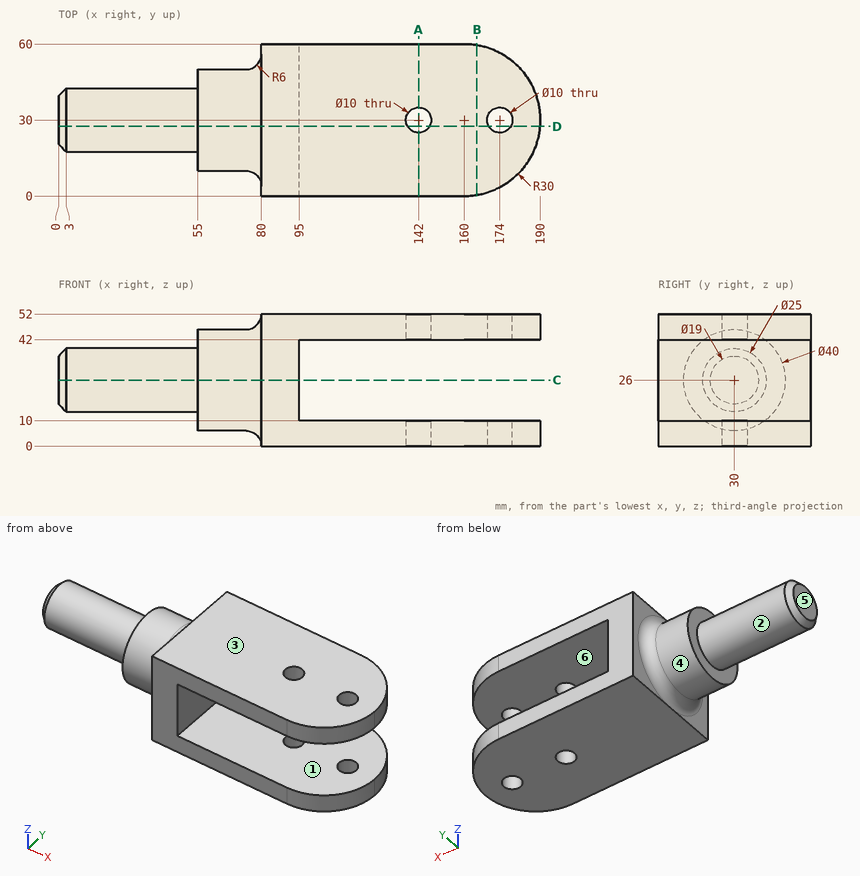
Design review of the part shown in the three views and the two pictorial views. Dimensions are in mm from the part's minimum x, y and z. A direction names the side the tool comes from. Round coordinates to 2 decimals unless told otherwise and drop trailing zeros. Write each loop counter-clockwise with the first axis right and the second up, starting at its lowest first coordinate (ties: lowest second). Pieces come first, ordered by that corner, then holes. Notation, with made-up numbers: (57, 47) - (110, 47) arc R25 cw to (110, 63) - close; hole circle Ø6 at (62.5, -23.75). An arc over 180 degrees is marked (long way). Write item = value, one per line. Start each with the question number.
1. Consider section D-D on y = 27.5. Give the number of separate pieces and of enclosed holes in the cut face, plus the area to 3 significant figures.
2. For the marked faces 1, 2 and 3, list the 3-axis set-ups (+Z, -Z, +X, -X, +Y, -Y) from which the entire face can be reached by the end or side of a thin tool; tool diameter is ignored.
3. Draft analysis for pull direction Z (two halves, no side actions). For the marked faces 4, 5 and 6, state which applies: released by +Z, released by -Z, zero draft, split by the parting line, or undercut.
4. Wall thickness on L1, parallel to X at y = 30, z = 45.75; L2, parallel to Z at x = 118, y = 19; L3, parallel to X at y = 30, z = 48: over which ranges is each line inside the solid? List them lowest first.
5. Consider section B-B on x = 165. State the section outline as (y, z) points, plus the area to 3 significant figures.
6. Consider section A-A on x = 142. State the section outline as (y, z) points.
7. For pin 1 Ø12 at (x, z) = (31, 16.5) entering from -Y; pin 2 Ø1.5 at (x, z) = (162, 5.5) entering from -Y; pin 3 Ø9.5 at (y, z) = (25.5, 30.5) entering from +X; pin 4 Ø10 at (x, z) = (125.5, 36.5) entering from +Y, all flat-tipped, find the tip position at first contact; note any pin that passes through.
8. Consider section C-C on z = 26. State the section outline as (x, y) points, plus the area to 3 significant figures.
Evaluation:
q1.separate_pieces = 5
q1.enclosed_holes = 0
q1.area = 4,680 mm2
q2.face_1 = +X, +Y, -Y
q2.face_2 = -X
q2.face_3 = +Z, +X, -X, +Y, -Y
q3.face_4 = split by the parting line
q3.face_5 = zero draft
q3.face_6 = undercut
q4.L1 = 55 to 137, 147 to 169, 179 to 190
q4.L2 = 0 to 10, 42 to 52
q4.L3 = 78.47 to 137, 147 to 169, 179 to 190
q5.outline = (0.42, 0) - (59.58, 0) - (59.58, 10) - (0.42, 10) - close; (0.42, 42) - (59.58, 42) - (59.58, 52) - (0.42, 52) - close
q5.area = 1,180 mm2
q6.outline = (0, 0) - (25, 0) - (25, 10) - (0, 10) - close; (0, 42) - (25, 42) - (25, 52) - (0, 52) - close; (35, 0) - (60, 0) - (60, 10) - (35, 10) - close; (35, 42) - (60, 42) - (60, 52) - (35, 52) - close
q7.pin_1 = 18
q7.pin_2 = 0.03
q7.pin_3 = 95
q7.pin_4 = through
q8.outline = (0, 20.5) - (3, 17.5) - (55, 17.5) - (55, 10) - (74, 10) arc R6 cw to (80, 4) - (80, 0) - (95, 0) - (95, 60) - (80, 60) - (80, 56) arc R6 cw to (74, 50) - (55, 50) - (55, 42.5) - (3, 42.5) - (0, 39.5) - close
q8.area = 3,280 mm2
